Geometry: see drawing. Coordinates: mm, zero at the bounding-box minimum. A direction names the side the tool comes from. Coordinates: 2 decimals unless noted, no trailing zeros. Write each loop counter-clockwise with the first axis right and the second up, starting at its lowest first coordinate (ties: lowest second). Pieces come first, ordered by that corner, then holes. Notation, with made-up numbers: M 74.25,4.5 L 102.25,4.5 A31 ccw 102.25,40.5 Z; hole C -13.5,88 d1. An arc over 180 degrees is marked long. One line per item, written item: value. Start each with the question number.
Item 1: Cut plane D-D, the plane x = 15. Output: boundary loops of the cut face in (y, z), then the cut area to 3 significant figures.
Item 2: Pin query (flat end, axial travel): P1, Ø6, axis at x = 16, y = 4.5, coming from the +Z side; P2, Ø8, axis at x = 8, z = 12.5, coming from the +Y side; P3, Ø5, axis at y = 2.5, z = 14.5, coming from the -X side. Return the tip coordinate at first contact, or that it passes through.
Item 3: Cut plane B-B, the plane x = 4. Output: boundary loops of the cut face in (y, z), then the cut area to 3 significant figures.
Item 4: Set-up query: the marked faces 1 and 2. Return all of +Z, -Z, +X, -X, +Y, -Y with unobstructed straight access to the full face (end or side cutting, diameter ignored); none if empty.
Item 5: Cut plane C-C, the plane z = 9.75. Output: boundary loops of the cut face in (x, y).
Item 6: Cut plane A-A, the plane y = 5. Output: boundary loops of the cut face in (x, z), then the cut area to 3 significant figures.
Item 7: Ray query, L1, parallel to Z at x = 18.75, y = 12.75; L2, parallel to Y at x = 5.5, z = 8.75; L3, parallel to X at y = 4.75, z = 13. Return the intervals inside material, ascending. Write a range as from..to.
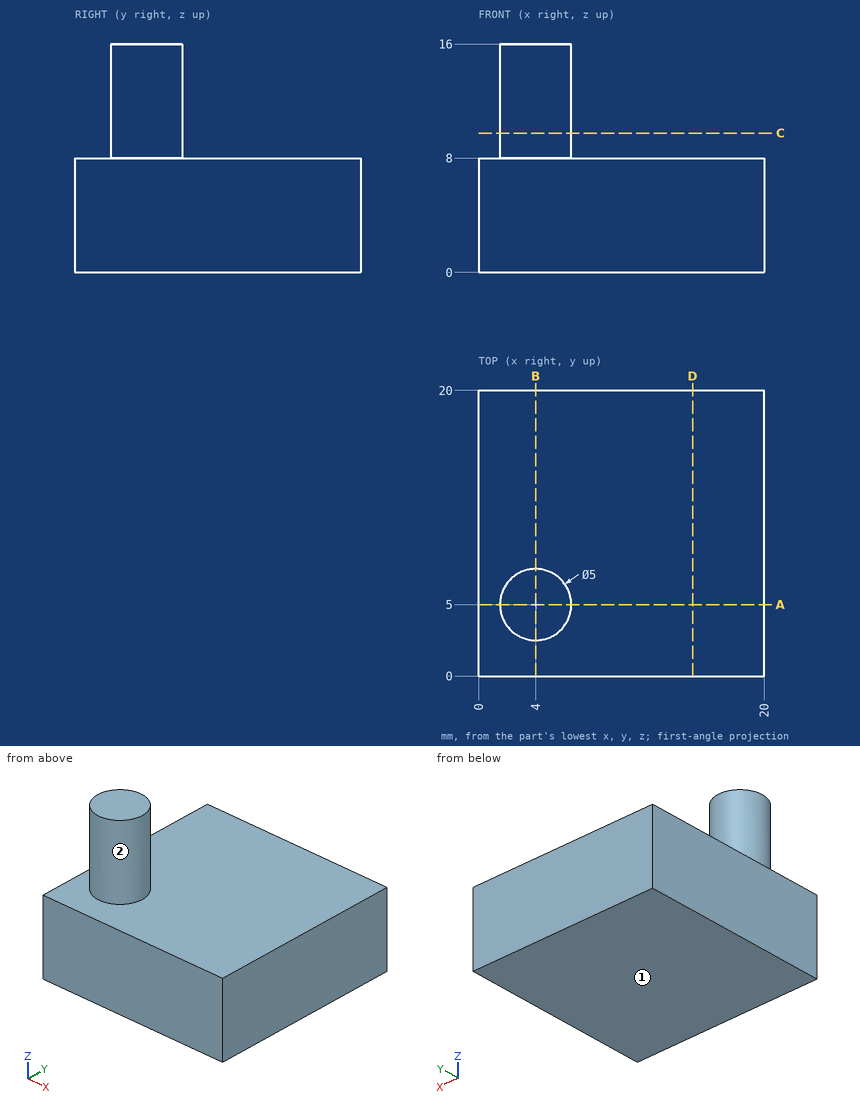
From the geometry:
1. outline: M 0,0 L 20,0 L 20,8 L 0,8 Z
1. area: 160 mm²
2. P1: stops at z = 8
2. P2: stops at y = 7.5
2. P3: stops at x = 1.5
3. outline: M 0,0 L 20,0 L 20,8 L 7.5,8 L 7.5,16 L 2.5,16 L 2.5,8 L 0,8 Z
3. area: 200 mm²
4. face 1: -Z, +X, -X, +Y, -Y
4. face 2: +Z
5. outline: C 4,5 d5
6. outline: M 0,0 L 20,0 L 20,8 L 6.5,8 L 6.5,16 L 1.5,16 L 1.5,8 L 0,8 Z
6. area: 200 mm²
7. L1: z = 0..8
7. L2: y = 3..7
7. L3: x = 1.51..6.49
